Here's how the part is built. I have some questions about the finished solid (model axes, mm). A direction names the side the tool comes from. Coordinates: 2 decimals unless noted, no trailing zeros. Write each loop counter-clockwise with the first axis right and the second up, starting at its lowest first coordinate (ties: lowest second). Pieces come first, ordered by that corner, then holes. Notation, with made-up numbers: M -2.75,6 L 41.25,6 A15 cw 41.25,33 Z; hole C 14,3.25 d3. An arc over 180 degrees is marked long. Use one line per item in the form item = value. Start each with the question number.
1. I want a section at A-A, the plane x = 68.5. List the corners of the cut face in (y, z) for me, plus the area to 3 significant figures.
2. Thinking about a two-plate mould opening in X: for faces 1 (the face through (58, 23, 16)), 2 (the face through (63, 19, 4)), 3 (the face through (39.5, 16, 17)), which applies, released by +X, released by -X, zero draft, split by the parting line, or undercut?
3. Please list where these lines run through material, in increasing order: line 1 along Y through (x, z) = (68.5, 19); line 2 along Y through (x, z) = (28.5, 10.5); line 3 along X through (y, z) = (11.25, 14.25). Write a range as [from, to].
4. On a 3-axis mill with a long thin cutter (end or side, diameter ignored), from which of +Z, -Z, +X, -X, +Y, -Y can I reach the whole of each face in a straight line? I mean faces 4 (the face through (31, 1, 17)), 5 (the face through (41, 9, 3)). Say none if no direction works.
5. I want a section at C-C, the plane x = 48.5. List the corners of the cut face in (y, z) for me.
6. I want a section at D-D, the plane z = 22.75. Count the separate pieces of the cut face and the enclosed holes in it, plus the area to 3 significant figures.
7. I want a section at B-B, the plane y = 16.5. List the corners of the cut face in (x, z) for me, plus the area to 3 significant figures.
8. I'm going to push flat-ended pins straight in: pin 1 Ø1.7 at (x, z) = (18, 15.5) entering from +Y; pin 2 Ø0.9 at (x, z) = (54, 5) entering from -Y; pin 3 Ø2.5 at (y, z) = (3, 5) entering from +X. Where does each tip first touch, or does it pass through?
from build123d import *

# Parameters (mm, degrees)
BOSS_EXTRUDE1_DEPTH = 30
SKETCH4_W           = 47
SKETCH4_H           = 3
CUT_EXTRUDE1_DEPTH  = 30
CUT_EXTRUDE2_DEPTH  = 3
SKETCH6_R           = 11.5
CUT_EXTRUDE3_DEPTH  = 3
CUT_EXTRUDE4_DEPTH  = 3
SKETCH8_R           = 1.75
CUT_EXTRUDE5_DEPTH  = 63
SKETCH9_R           = 1.25
CUT_EXTRUDE6_DEPTH  = 63
SKETCH11_R          = 1.75
CUT_EXTRUDE7_DEPTH  = 63
CUT_EXTRUDE8_START  = -30
CUT_EXTRUDE8_DEPTH  = 30
CUT_EXTRUDE12_DEPTH = 3
SKETCH26_W          = 13.519432365
SKETCH26_H          = 72.724713812
CUT_EXTRUDE18_DEPTH = 3
SKETCH21_W          = 40
SKETCH21_H          = 3
CUT_EXTRUDE16_DEPTH = 27
SKETCH19_W          = 40
SKETCH19_H          = 3
CUT_EXTRUDE15_DEPTH = 77
SKETCH27_W          = 110.290259741
SKETCH27_H          = 28.330573593
CUT_EXTRUDE19_DEPTH = 98.765024421


# Read off the part's stored shape, not the designer's step: Cut-Extrude8
with BuildPart() as part:
    # Sketch2 → Boss-Extrude1 (new body)
    with BuildSketch(Plane.XY):
        Polygon((2, 0), (0, 0), (1, -1.732050808), align=None)
        Polygon((4, 0), (2, 0), (3, -1.732050808), align=None)
        Polygon((6, 0), (4, 0), (5, -1.732050808), align=None)
        Polygon((8, 0), (6, 0), (7, -1.732050808), align=None)
        Polygon((10, 0), (8, 0), (9, -1.732050808), align=None)
        Polygon((12, 0), (10, 0), (11, -1.732050808), align=None)
        Polygon((14, 0), (12, 0), (13, -1.732050808), align=None)
        Polygon((16, 0), (14, 0), (15, -1.732050808), align=None)
        Polygon((18, 0), (16, 0), (17, -1.732050808), align=None)
        Polygon((20, 0), (18, 0), (19, -1.732050808), align=None)
        Polygon((22, 0), (20, 0), (21, -1.732050808), align=None)
        Polygon((24, 0), (22, 0), (23, -1.732050808), align=None)
        Polygon((25, -1.732050808), (26, 0), (24, 0), align=None)
        Polygon((27, -1.732050808), (28, 0), (26, 0), align=None)
        Polygon((29, -1.732050808), (30, 0), (28, 0), align=None)
        Polygon((31, -1.732050808), (32, 0), (30, 0), align=None)
        Polygon((33, -1.732050808), (34, 0), (32, 0), align=None)
        Polygon((35, -1.732050808), (36, 0), (34, 0), align=None)
        Polygon((37, -1.732050808), (38, 0), (36, 0), align=None)
        Polygon((39, -1.732050808), (40, 0), (38, 0), align=None)
        Polygon((75.5, 23), (75.5, 0), (0, 0), (40, 23), align=None)
        with BuildLine():
            ThreePointArc((75.5, 0), (87, 11.5), (75.5, 23))
            Line((75.5, 23), (75.5, 0))
        make_face()
    extrude(amount=BOSS_EXTRUDE1_DEPTH)

    # Sketch4 → Cut-Extrude1 (cut)
    with BuildSketch(Plane.XZ):
        with Locations((63.5, 1.5)):
            Rectangle(SKETCH4_W, SKETCH4_H)
    extrude(amount=-CUT_EXTRUDE1_DEPTH, mode=Mode.SUBTRACT)

    # Sketch5 → Cut-Extrude2 (cut)
    with BuildSketch(Plane(origin=(0, 0, 3), x_dir=(-1, 0, 0), z_dir=(0, 0, -1))):
        with BuildLine():
            Line((-44.5, 15.5), (-100.316269326, 15.5))
            Line((-100.316269326, 15.5), (-100.316269326, 7.5))
            Line((-100.316269326, 7.5), (-44.5, 7.5))
            ThreePointArc((-44.5, 7.5), (-40.5, 11.5), (-44.5, 15.5))
        make_face()
    extrude(amount=-CUT_EXTRUDE2_DEPTH, mode=Mode.SUBTRACT)

    # Sketch6 → Cut-Extrude3 (cut)
    with BuildSketch(Plane(origin=(0, 0, 3), x_dir=(-1, 0, 0), z_dir=(0, 0, -1))):
        with Locations((-75.5, 11.5)):
            Circle(SKETCH6_R)
    extrude(amount=-CUT_EXTRUDE3_DEPTH, mode=Mode.SUBTRACT)

    # Sketch7 → Cut-Extrude4 (cut)
    with BuildSketch(Plane(origin=(0, 0, 3), x_dir=(-1, 0, 0), z_dir=(0, 0, -1))):
        with BuildLine():
            Line((-64.718070674, 7.5), (-64.718070674, 0))
            Line((-64.718070674, 0), (-75.5, 0))
            ThreePointArc((-75.5, 0), (-68.933037232, 2.059396206), (-64.718070674, 7.5))
        make_face()
    extrude(amount=-CUT_EXTRUDE4_DEPTH, mode=Mode.SUBTRACT)

    # Sketch8 → Cut-Extrude5 (cut)
    with BuildSketch(Plane(origin=(0, 0, 6), x_dir=(-1, 0, 0), z_dir=(0, 0, -1))):
        with Locations((-75.5, 11.5)):
            Circle(SKETCH8_R)
    extrude(amount=-CUT_EXTRUDE5_DEPTH, mode=Mode.SUBTRACT)

    # Sketch9 → Cut-Extrude6 (cut)
    with BuildSketch(Plane(origin=(0, 0, 6), x_dir=(-1, 0, 0), z_dir=(0, 0, -1))):
        with Locations((-68.5, 11.5)):
            Circle(SKETCH9_R)
        with Locations((-82.5, 11.5)):
            Circle(SKETCH9_R)
    extrude(amount=-CUT_EXTRUDE6_DEPTH, mode=Mode.SUBTRACT)

    # Sketch11 → Cut-Extrude7 (cut)
    with BuildSketch(Plane(origin=(0, 0, 6), x_dir=(-1, 0, 0), z_dir=(0, 0, -1))):
        with Locations((-44.5, 11.5)):
            Circle(SKETCH11_R)
    extrude(amount=-CUT_EXTRUDE7_DEPTH, mode=Mode.SUBTRACT)

    # Cut-Extrude8 outline → Cut-Extrude8 (cut)
    with BuildSketch(Plane(origin=(0, 0, 0), x_dir=(-1, 0, 0), z_dir=(0, 0, -1)).offset(CUT_EXTRUDE8_START)):
        with BuildLine():
            ThreePointArc((-32.629244175, 14.144182994), (-31.629244953, 15.877998297), (-32.632301926, 17.610046408))
            Line((-32.632301926, 17.610046408), (-36.503057751, 19.835731008))
            ThreePointArc((-36.503057751, 19.835731008), (-38.501527709, 19.833086287), (-39.5, 18.101918401))
            Line((-39.5, 18.101918401), (-39.5, 13.641451884))
            ThreePointArc((-39.5, 13.641451884), (-38.5, 11.909401077), (-36.5, 11.909401077))
            Line((-36.5, 11.909401077), (-32.629244175, 14.144182994))
        make_face()
        with BuildLine():
            ThreePointArc((-7.49052939, 1), (-6.524375597, 1.742033241), (-6.992058265, 2.866906303))
            Line((-6.992058265, 2.866906303), (-8.609059399, 3.796681955))
            ThreePointArc((-8.609059399, 3.796681955), (-9.106957749, 3.929775488), (-9.605008237, 3.797252409))
            ThreePointArc((-9.605008237, 3.797252409), (-10.300350282, 2.110050397), (-8.851923789, 1))
            Line((-8.851923789, 1), (-7.49052939, 1))
        make_face()
        with BuildLine():
            ThreePointArc((-24.565011822, 9.507249391), (-23.5650126, 11.241064694), (-24.568069573, 12.973112805))
            Line((-24.568069573, 12.973112805), (-26.524452009, 14.098032706))
            ThreePointArc((-26.524452009, 14.098032706), (-29.021218869, 14.763499245), (-31.516807631, 14.09362821))
            Line((-31.516807631, 14.09362821), (-37, 10.927905619))
            ThreePointArc((-37, 10.927905619), (-38.830127019, 9.0977786), (-39.5, 6.5977786))
            Line((-39.5, 6.5977786), (-39.5, 4.348631561))
            ThreePointArc((-39.5, 4.348631561), (-38.5, 2.616580754), (-36.5, 2.616580754))
            Line((-36.5, 2.616580754), (-24.565011822, 9.507249391))
        make_face()
        with BuildLine():
            ThreePointArc((-21.101923789, 3.799038106), (-21.800812528, 2.111771433), (-20.351923789, 1))
            Line((-20.351923789, 1), (-16.989745962, 1))
            ThreePointArc((-16.989745962, 1), (-15.695650737, 1.170370869), (-14.489745962, 1.669872981))
            Line((-14.489745962, 1.669872981), (-12.715894213, 2.694006766))
            ThreePointArc((-12.715894213, 2.694006766), (-11.717324154, 4.350441969), (-12.587876643, 6.077595149))
            ThreePointArc((-12.587876643, 6.077595149), (-14.991941557, 6.624711226), (-17.365185047, 5.956445224))
            Line((-17.365185047, 5.956445224), (-21.101923789, 3.799038106))
        make_face()
        with BuildLine():
            ThreePointArc((-33.251923789, 3.799038106), (-33.950812528, 2.111771433), (-32.501923789, 1))
            Line((-32.501923789, 1), (-28.489745962, 1))
            ThreePointArc((-28.489745962, 1), (-27.195650737, 1.170370869), (-25.989745962, 1.669872981))
            Line((-25.989745962, 1.669872981), (-18.477621591, 6.007000009))
            ThreePointArc((-18.477621591, 6.007000009), (-17.477623561, 7.73624352), (-18.472763157, 9.468287505))
            ThreePointArc((-18.472763157, 9.468287505), (-20.964215142, 10.126554039), (-23.452575278, 9.456694606))
            Line((-23.452575278, 9.456694606), (-33.251923789, 3.799038106))
        make_face()
    extrude(amount=CUT_EXTRUDE8_DEPTH, mode=Mode.SUBTRACT)

    # Sketch15 → Cut-Extrude12 (cut)
    with BuildSketch(Plane(origin=(0, 0, 3), x_dir=(-1, 0, 0), z_dir=(0, 0, -1))):
        with BuildLine():
            Line((-75.5, 23), (-70.601020514, 23))
            ThreePointArc((-70.601020514, 23), (-66.32756197, 19.992136397), (-63.657280718, 15.5))
            Line((-63.657280718, 15.5), (-64.718070674, 15.5))
            ThreePointArc((-64.718070674, 15.5), (-68.933037232, 20.940603794), (-75.5, 23))
        make_face()
    extrude(amount=-CUT_EXTRUDE12_DEPTH, mode=Mode.SUBTRACT)


with BuildPart() as body_2:
    # Mirror6: mirrored copy
    add(part.part.mirror(Plane(origin=(0, -5, 0), x_dir=(0, 0, 1), z_dir=(0, -1, 0))))


with BuildPart() as cut_extrude18_tool:
    # Sketch26 → Cut-Extrude18 (new body)
    with BuildSketch(Plane(origin=(0, 0, 3), x_dir=(-1, 0, 0), z_dir=(0, 0, -1))):
        with Locations((-69.759716183, -4.516968795)):
            Rectangle(SKETCH26_W, SKETCH26_H)
    extrude(amount=-CUT_EXTRUDE18_DEPTH)


with BuildPart() as part_1:
    add(part.part)

    # Cut-Extrude18: cut by cut_extrude18_tool
    add(cut_extrude18_tool.part, mode=Mode.SUBTRACT)

    # Sketch21 → Cut-Extrude16 (cut)
    with BuildSketch(Plane(origin=(0, 23, 0), x_dir=(1, 0, 0), z_dir=(0, 1, 0))):
        with Locations((20, -1.5)):
            Rectangle(SKETCH21_W, SKETCH21_H)
    extrude(amount=-CUT_EXTRUDE16_DEPTH, mode=Mode.SUBTRACT)


with BuildPart() as body_2_1:
    add(body_2.part)

    # Cut-Extrude18: cut by cut_extrude18_tool
    add(cut_extrude18_tool.part, mode=Mode.SUBTRACT)

    # Sketch19 → Cut-Extrude15 (cut)
    with BuildSketch(Plane.XZ.offset(33)):
        with Locations((20, 1.5)):
            Rectangle(SKETCH19_W, SKETCH19_H)
    extrude(amount=-CUT_EXTRUDE15_DEPTH, mode=Mode.SUBTRACT)

    # Sketch27 → Cut-Extrude19 (cut, through all)
    with BuildSketch(Plane.XY):
        with Locations((42.931493507, -21.344561689)):
            Rectangle(SKETCH27_W, SKETCH27_H)
    extrude(amount=CUT_EXTRUDE19_DEPTH, mode=Mode.SUBTRACT)


solid = part_1.part
Answer list:
q1.outline = M 0,6 L 10.25,6 L 10.25,30 L 0,30 Z; M 12.75,6 L 23,6 L 23,30 L 12.75,30 Z
q1.area = 492 mm²
q2.face_1 = zero draft
q2.face_2 = released by +X
q2.face_3 = undercut
q3.line_1 = [0, 10.25], [12.75, 23]
q3.line_2 = [-0.87, 1], [6.54, 7.24], [14.74, 16.39]
q3.line_3 = [19.57, 23.57], [36.44, 42.77], [46.23, 67.28], [69.72, 73.77], [77.23, 81.28], [83.72, 87]
q4.face_4 = +Z, -Z
q4.face_5 = -Z, +X, -X, +Y, -Y
q5.outline = M 0,3 L 7.5,3 L 7.5,6 L 15.5,6 L 15.5,3 L 23,3 L 23,30 L 0,30 Z
q6.separate_pieces = 1
q6.enclosed_holes = 9
q6.area = 1,200 mm²
q7.outline = M 28.7,3 L 31.73,3 L 31.73,30 L 28.7,30 Z; M 39.5,3 L 63,3 L 63,6 L 85.86,6 L 85.86,30 L 39.5,30 Z
q7.area = 1,260 mm²
q8.pin_1 = 10.84
q8.pin_2 = 0
q8.pin_3 = 84
